Read the model definition and answer for the solid it produces. Units are mm, in the model's axes. A direction names the side the tool comes from. Coordinates: 2 decimals unless noted, no trailing zeros. Loops run counter-clockwise (first coordinate to the right, second up) from the corner with the lowest first, then second, coordinate; pieces in that order, holes last.
Q1. Section C-C (y = 5.55) is taken. Give the vertices of the cut face in (x, z).
Q2. Straight lines are drawn through the part: line 1 (X direction, y = 1.45, z = 0); line 2 (X direction, y = 2.8, z = 0); line 3 (Z direction, x = -5.5, y = 4.75). For each, find the intervals that lie inside material, in ascending order.
Q3. Section A-A (x = -5) is taken. Give the vertices of the cut face in (y, z), then the cut area to 3 significant figures.
Q4. Flat-ended cylindrical pins translate along their axes: P1, Ø1.5, axis at y = 4, z = 5.5, coming from the +X side; P2, Ø1, axis at x = -4, y = 1.5, coming from the -Z side. Find the tip coordinate at first contact, or state that the pin passes through.
Q5. Section D-D (z = 5.25) is taken. Give the vertices of the cut face in (x, y).
Q6. Which of the six approach directions +Z, -Z, +X, -X, +Y, -Y give full straight-line access (tool end or side, diameter ignored) to faces 5 (the face through (0, 0, 0)), 6 (the face through (-9.76, 3.97, -2.17))?
Q7. The mould has two halves that part along Z. Classify faces 1 (the face through (0, 6, 0)), 2 (the face through (3.94, 2.96, -0.35)), 3 (the face through (-10.74, 0.99, 2.38)), 4 (the face through (-7.06, 2.96, -0.35)): pulls with the +Z half, pulls with the -Z half, needs draft (parallel to the pull), parting line crosses it, or undercut.
Q8. Section B-B (x = 0) is taken. Give the vertices of the cut face in (y, z).
from build123d import *

# Parameters (mm, degrees)
SKETCH1_R           = 10
BOSS_EXTRUDE1_DEPTH = 6
SKETCH4_R           = 11
BOSS_EXTRUDE2_DEPTH = 2
SKETCH3_R           = 1.6
CUT_EXTRUDE2_DEPTH  = 15


with BuildPart() as part:
    # Sketch1 → Boss-Extrude1 (new body)
    with BuildSketch(Plane(origin=(0, 0, 0), x_dir=(1, 0, 0), z_dir=(0, 1, 0))):
        with Locations(Location((0, 0, 0), (0, 0, 270))):
            Circle(SKETCH1_R)
    extrude(amount=BOSS_EXTRUDE1_DEPTH)

    # Sketch4 → Boss-Extrude2 (add)
    with BuildSketch(Plane.XZ):
        with Locations(Location((0, 0, 0), (0, 0, 270))):
            Circle(SKETCH4_R)
    extrude(amount=-BOSS_EXTRUDE2_DEPTH)

    # Sketch3 → Cut-Extrude2 (cut)
    with BuildSketch(Plane(origin=(0, 0, 0), x_dir=(1, 0, 0), z_dir=(0, 1, 0))):
        with Locations(Location((-5.5, 0, 0), (0, 0, 270))):
            Circle(SKETCH3_R)
        with Locations(Location((5.5, 0, 0), (0, 0, 270))):
            Circle(SKETCH3_R)
    extrude(amount=CUT_EXTRUDE2_DEPTH, mode=Mode.SUBTRACT)


solid = part.part
Numbers:
1. outline: circle Ø20 at (0, 0); hole circle Ø3.2 at (-5.5, 0); hole circle Ø3.2 at (5.5, 0)
2. line 1: x = -11 to -7.1, -3.9 to 3.9, 7.1 to 11
2. line 2: x = -10 to -7.1, -3.9 to 3.9, 7.1 to 10
2. line 3: z = -8.35 to -1.6, 1.6 to 8.35
3. outline: (0, -9.8) - (2, -9.8) - (2, -8.66) - (6, -8.66) - (6, -1.52) - (0, -1.52) - close; (0, 1.52) - (6, 1.52) - (6, 8.66) - (2, 8.66) - (2, 9.8) - (0, 9.8) - close
3. area: 90.2 mm2
4. P1: stops at x = 8.8
4. P2: stops at z = -10.43
5. outline: (-9.67, 0) - (9.67, 0) - (9.67, 2) - (8.51, 2) - (8.51, 6) - (-8.51, 6) - (-8.51, 2) - (-9.67, 2) - close
6. face 5: +Z, -Z, +X, -X, -Y
6. face 6: +Y
7. face 1: needs draft
7. face 2: undercut
7. face 3: parting line crosses it
7. face 4: undercut
8. outline: (0, -11) - (2, -11) - (2, -10) - (6, -10) - (6, 10) - (2, 10) - (2, 11) - (0, 11) - close
